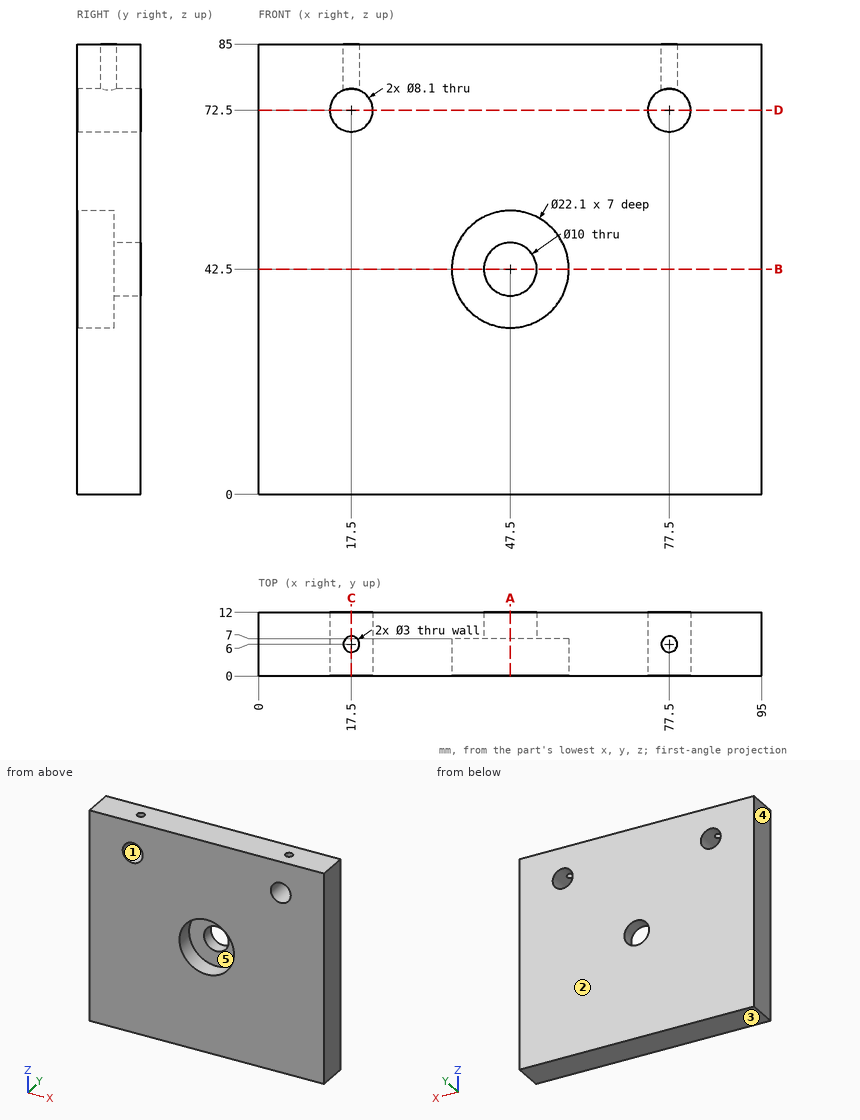
Verification items for this drawing (mm, ordinates from the low corner). A direction names the side the tool comes from. Coordinates: 2 decimals unless noted, no trailing zeros. Write each loop counter-clockwise with the first axis right and the second up, starting at its lowest first coordinate (ties: lowest second). Pieces come first, ordered by that corner, then holes. Notation, with made-up numbers: (23, 49.5) -> (67, 49.5) arc R24 cw to (67, 62.5) -> close; hole circle Ø3 at (79, 52.25). An arc over 180 degrees is marked (long way). One line per item, written item: value. Start each with the question number.
Q1. Go/stop test with flat-tipped pins: P1, Ø1.5, axis at x = 85, y = 3, coming from the -Z side; P2, Ø1.5, axis at x = 44.5, z = 46, coming from the -Y side. Record where each tip stops, or that it passes through.
Q2. Cross-section at C-C on x = 17.5. Enter the section's corners in (y, z).
Q3. Access from +Z, -Z, +X, -X, +Y, -Y to the whole of each face (thin tool, end or side, straight path). Record for the marked faces 4 and 5.
Q4. Thickness scan on L1, parallel to X at y = 8, z = 72.5; L2, parallel to Z at x = 17.5, y = 5.75; L3, parallel to Z at x = 43.5, y = 3. Record the ranges inside material, lowest first. Write a range as from..to.
Q5. Mould release check, pull along Z, two halves, no side actions. Record for the marked faces 1, 2 and 3: pulls with the +Z half, pulls with the -Z half, needs draft (parallel to the pull), parting line crosses it, or undercut.
Q6. Cross-section at A-A on x = 47.5. Enter the section's corners in (y, z).
Q7. Cross-section at D-D on z = 72.5. Enter the section's corners in (x, y).
Q8. Cross-section at B-B on z = 42.5. Enter the section's corners in (x, y), and give its area (3 significant figures).
Checked values:
1. P1: stops at z = 0
1. P2: stops at y = 7
2. outline: (0, 0) -> (12, 0) -> (12, 68.45) -> (0, 68.45) -> close; (0, 76.55) -> (4.5, 76.55) -> (4.5, 85) -> (0, 85) -> close; (7.5, 76.55) -> (12, 76.55) -> (12, 85) -> (7.5, 85) -> close
3. face 4: +Z, -Z, -X, +Y, -Y
3. face 5: -Y
4. L1: x = 0..13.45, 21.55..73.45, 81.55..95
4. L2: z = 0..68.45
4. L3: z = 0..32.2, 52.8..85
5. face 1: undercut
5. face 2: needs draft
5. face 3: pulls with the -Z half
6. outline: (0, 0) -> (12, 0) -> (12, 37.5) -> (7, 37.5) -> (7, 31.45) -> (0, 31.45) -> close; (0, 53.55) -> (7, 53.55) -> (7, 47.5) -> (12, 47.5) -> (12, 85) -> (0, 85) -> close
7. outline: (0, 0) -> (13.45, 0) -> (13.45, 12) -> (0, 12) -> close; (21.55, 0) -> (73.45, 0) -> (73.45, 12) -> (21.55, 12) -> close; (81.55, 0) -> (95, 0) -> (95, 12) -> (81.55, 12) -> close
8. outline: (0, 0) -> (36.45, 0) -> (36.45, 7) -> (42.5, 7) -> (42.5, 12) -> (0, 12) -> close; (52.5, 7) -> (58.55, 7) -> (58.55, 0) -> (95, 0) -> (95, 12) -> (52.5, 12) -> close
8. area: 935 mm²
